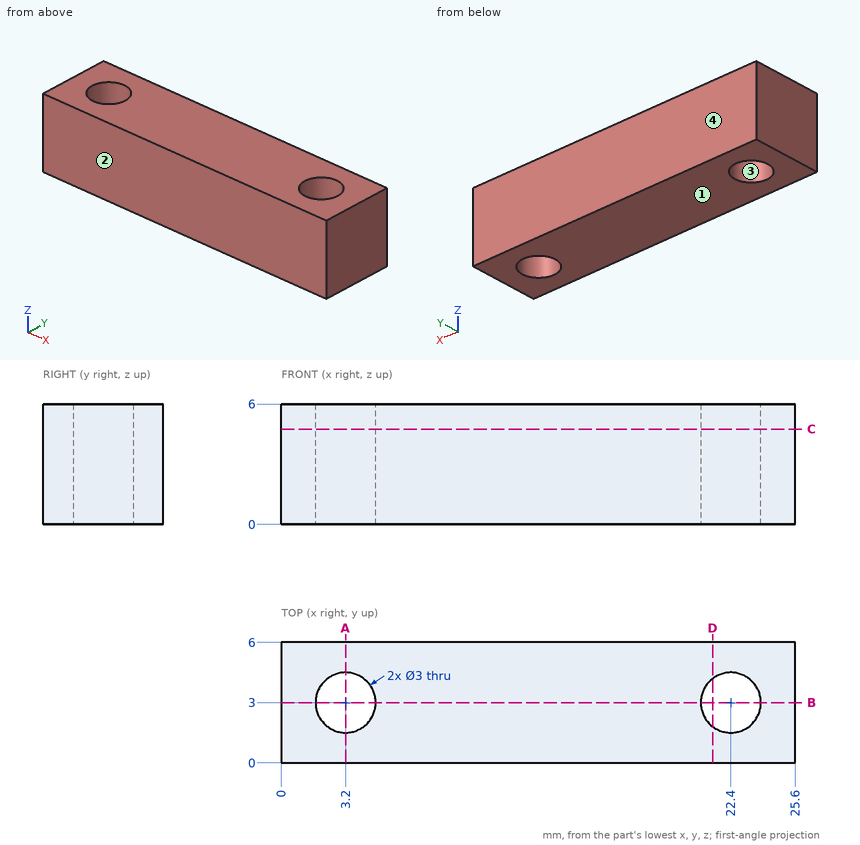
Drawing for the job (mm, zero at the part's lowest x, y, z). Round coordinates to 2 decimals unless told otherwise and drop trailing zeros. Order: outer loops, then holes, each group sorted by start corner. A loop starts at its lowest first (then second) coordinate and runs counter-clockwise, first axis right, second up. Notation, with made-up numbers: M 81,20 L 111,20 A17 ccw 111,36 Z; hole C -6,-4.75 d10. An arc over 180 degrees is marked long. Use one line per item in the form item = value.
Q1. Saw through at D-D on x = 21.5. Give the cut face in (y, z).
Recorded:
outline = M 0,0 L 1.8,0 L 1.8,6 L 0,6 Z; M 4.2,0 L 6,0 L 6,6 L 4.2,6 Z
Q2. Flat gauge pin, fed straight in: P1, Ø1.8, axis at x = 3.2, y = 3, coming from the -Z side. Where does the tip first touch, or does it go through?
Recorded:
P1 = through
Q3. Saw through at B-B on y = 3. Give the cut face in (x, z).
Recorded:
outline = M 0,0 L 1.7,0 L 1.7,6 L 0,6 Z; M 4.7,0 L 20.9,0 L 20.9,6 L 4.7,6 Z; M 23.9,0 L 25.6,0 L 25.6,6 L 23.9,6 Z
Q4. Probe L1, parallel to Y at x = 22.4, z = 1.7; L2, parallel to X at y = 3.8, z = 1.9; L3, parallel to Y at x = 21.75, z = 0.8. List the from-to ranges inside material, lowest first.
Recorded:
L1 = 0 to 1.5, 4.5 to 6
L2 = 0 to 1.93, 4.47 to 21.13, 23.67 to 25.6
L3 = 0 to 1.65, 4.35 to 6
Q5. Two-plate mould, pull along Y, no slides. Class the marked faces 1, 2, 3 and 4: +Y half, -Y half, draft (parallel to the pull), parting line (faces both ways), or undercut.
Recorded:
face_1 = draft
face_2 = -Y half
face_3 = undercut
face_4 = +Y half
Q6. Saw through at A-A on x = 3.2. Give the cut face in (y, z), then the cut area to 3 significant figures.
Recorded:
outline = M 0,0 L 1.5,0 L 1.5,6 L 0,6 Z; M 4.5,0 L 6,0 L 6,6 L 4.5,6 Z
area = 18.0 mm^2
Q7. Saw through at C-C on z = 4.75. Give the cut face in (x, y).
Recorded:
outline = M 0,0 L 25.6,0 L 25.6,6 L 0,6 Z; hole C 3.2,3 d3; hole C 22.4,3 d3
